The listing builds one solid part. Answer for the finished solid, in the listing's coordinates (mm). A direction names the side the tool comes from. Give positions to 0.01 mm unless a question says otherwise; leave off trailing zeros. Order: outer loops, then holes, each group sorted by start corner. A loop starts at its lowest first (then second) coordinate and runs counter-clockwise, first axis right, second up.
```python
from build123d import *

# Parameters (mm, degrees)
SKETCH1_W                     = 96.825
SKETCH1_H                     = 96.825
BOSS_EXTRUDE1_DEPTH           = 4.7625
FILLET1_R                     = 4
CSK_FOR_M3_SFHCS2_D           = 3.4
CSK_FOR_M3_SFHCS2_CSINK_D     = 6.72
CSK_FOR_M3_SFHCS2_CSINK_ANGLE = 90
CSK_FOR_M3_SFHCS1_D           = 3.4
CSK_FOR_M3_SFHCS1_DEPTH       = 35
CSK_FOR_M3_SFHCS1_CSINK_D     = 6.72
CSK_FOR_M3_SFHCS1_CSINK_ANGLE = 90
CSK_FOR_M3_SFHCS1_TIP         = 1.021463052
M3X0_5_TAPPED_HOLE1_D         = 2.5
M3X0_5_TAPPED_HOLE1_DEPTH     = 10
M3X0_5_TAPPED_HOLE1_TIP       = 0.751075774
M3X0_5_TAPPED_HOLE2_D         = 2.5
M3X0_5_TAPPED_HOLE2_DEPTH     = 10
M3X0_5_TAPPED_HOLE2_TIP       = 0.751075774
M3X0_5_TAPPED_HOLE3_D         = 2.5
M3X0_5_TAPPED_HOLE3_DEPTH     = 10
M3X0_5_TAPPED_HOLE3_TIP       = 0.751075774
M3X0_5_TAPPED_HOLE4_D         = 2.5
M3X0_5_TAPPED_HOLE4_DEPTH     = 10
M3X0_5_TAPPED_HOLE4_TIP       = 0.751075774


with BuildPart() as part:
    # Sketch1 → Boss-Extrude1 (new body, symmetric)
    with BuildSketch(Plane(origin=(0, 0, 0), x_dir=(1, 0, 0), z_dir=(0, 1, 0))):
        Rectangle(SKETCH1_W, SKETCH1_H)
    extrude(amount=BOSS_EXTRUDE1_DEPTH, both=True)

    # Fillet1
    fillet1_edges = [part.edges().sort_by_distance(p)[0] for p in [
        (-48.4125, 0, -48.4125),
        (48.4125, 0, -48.4125),
        (48.4125, 0, 48.4125),
        (-48.4125, 0, 48.4125),
    ]]
    fillet(fillet1_edges, radius=FILLET1_R)

    # CSK for M3 SFHCS2 (through all)
    with Locations(Plane.XZ.offset(4.7625)):
        with Locations((-40, 0), (0, -40), (40, 0), (0, 40)):
            CounterSinkHole(CSK_FOR_M3_SFHCS2_D / 2, CSK_FOR_M3_SFHCS2_CSINK_D / 2, counter_sink_angle=CSK_FOR_M3_SFHCS2_CSINK_ANGLE)

    # CSK for M3 SFHCS1
    with Locations(Plane(origin=(0, 4.7625, 0), x_dir=(1, 0, 0), z_dir=(0, 1, 0))):
        with Locations((-44.4125, 44.4125), (44.4125, 44.4125), (44.4125, -44.4125), (-44.4125, -44.4125)):
            CounterSinkHole(CSK_FOR_M3_SFHCS1_D / 2, CSK_FOR_M3_SFHCS1_CSINK_D / 2, depth=CSK_FOR_M3_SFHCS1_DEPTH, counter_sink_angle=CSK_FOR_M3_SFHCS1_CSINK_ANGLE)
            with Locations((0, 0, -(CSK_FOR_M3_SFHCS1_DEPTH + CSK_FOR_M3_SFHCS1_TIP / 2))):  # 118° drill point
                Cone(0, CSK_FOR_M3_SFHCS1_D / 2, CSK_FOR_M3_SFHCS1_TIP, mode=Mode.SUBTRACT)

    # M3x0.5 Tapped Hole1
    with Locations(Plane.XY.offset(48.4125)):
        with Locations((-30, 0), (30, 0)):
            Hole(M3X0_5_TAPPED_HOLE1_D / 2, depth=M3X0_5_TAPPED_HOLE1_DEPTH)
            with Locations((0, 0, -(M3X0_5_TAPPED_HOLE1_DEPTH + M3X0_5_TAPPED_HOLE1_TIP / 2))):  # 118° drill point
                Cone(0, M3X0_5_TAPPED_HOLE1_D / 2, M3X0_5_TAPPED_HOLE1_TIP, mode=Mode.SUBTRACT)

    # M3x0.5 Tapped Hole2
    with Locations(Plane.ZY.offset(48.4125)):
        with Locations((-30, 0), (30, 0)):
            Hole(M3X0_5_TAPPED_HOLE2_D / 2, depth=M3X0_5_TAPPED_HOLE2_DEPTH)
            with Locations((0, 0, -(M3X0_5_TAPPED_HOLE2_DEPTH + M3X0_5_TAPPED_HOLE2_TIP / 2))):  # 118° drill point
                Cone(0, M3X0_5_TAPPED_HOLE2_D / 2, M3X0_5_TAPPED_HOLE2_TIP, mode=Mode.SUBTRACT)

    # M3x0.5 Tapped Hole3
    with Locations(Plane(origin=(0, 0, -48.4125), x_dir=(-1, 0, 0), z_dir=(0, 0, -1))):
        with Locations((-30, 0), (30, 0)):
            Hole(M3X0_5_TAPPED_HOLE3_D / 2, depth=M3X0_5_TAPPED_HOLE3_DEPTH)
            with Locations((0, 0, -(M3X0_5_TAPPED_HOLE3_DEPTH + M3X0_5_TAPPED_HOLE3_TIP / 2))):  # 118° drill point
                Cone(0, M3X0_5_TAPPED_HOLE3_D / 2, M3X0_5_TAPPED_HOLE3_TIP, mode=Mode.SUBTRACT)

    # M3x0.5 Tapped Hole4
    with Locations(Plane(origin=(48.4125, 0, 0), x_dir=(0, 0, -1), z_dir=(1, 0, 0))):
        with Locations((-30, 0), (30, 0)):
            Hole(M3X0_5_TAPPED_HOLE4_D / 2, depth=M3X0_5_TAPPED_HOLE4_DEPTH)
            with Locations((0, 0, -(M3X0_5_TAPPED_HOLE4_DEPTH + M3X0_5_TAPPED_HOLE4_TIP / 2))):  # 118° drill point
                Cone(0, M3X0_5_TAPPED_HOLE4_D / 2, M3X0_5_TAPPED_HOLE4_TIP, mode=Mode.SUBTRACT)


solid = part.part
```
1) Find section A-A (z = 0). Write down the section's boundary in (x, y).
Geometry says:
outline: (-48.41, -4.76) - (-43.36, -4.76) - (-41.7, -3.1) - (-41.7, 4.76) - (-48.41, 4.76) - close; (-38.3, -3.1) - (-36.64, -4.76) - (36.64, -4.76) - (38.3, -3.1) - (38.3, 4.76) - (-38.3, 4.76) - close; (41.7, -3.1) - (43.36, -4.76) - (48.41, -4.76) - (48.41, 4.76) - (41.7, 4.76) - close
2) For a pull along Z with two mould halves and no side action, classify faces 1 (the flat face through (48.412, 0, 1)), 2 (the cylindrical face through (-47.27, -0.07, -47.21)), 3 (the flat face through (-1, 0, 48.412)), 4 (the conical face through (-37.79, -0.08, -29.8)) as +Z half, -Z half, draft (parallel to the pull), parting line (faces both ways), or undercut.
Geometry says:
face 1: draft
face 2: -Z half
face 3: +Z half
face 4: undercut
3) Given P1, Ø2, axis at x = 30, y = 0, coming from the +Z side; P2, Ø2, axis at x = -30, y = 0, coming from the -Z side; P3, Ø1.5, axis at y = 0, z = 30, coming from the +X side, each flat-ended and moving along its own axis, determine where each tip first touches the part or whether it passes through.
Geometry says:
P1: stops at z = 38.26
P2: stops at z = -38.26
P3: stops at x = 38.11
4) Straight lines are drawn through the part: probe 1 along X at (y, z) = (0, 42.25); probe 2 along Y at (x, z) = (42, -30); probe 3 along Z at (x, y) = (40, -0.75). For each, find the intervals that lie inside material, in ascending order.
Geometry says:
probe 1: x = -48.41 to -31.25, -28.75 to 28.75, 31.25 to 48.41
probe 2: y = -4.76 to -1.25, 1.25 to 4.76
probe 3: z = -48.41 to -31, -29 to -1.7, 1.7 to 29, 31 to 48.41
5) A tool of negligible diameter and unlimited length cuts with its end or side. For faces 5 (the cylindrical face through (31.155, -0.479, -43.342)), 6 (the cylindrical face through (-43.342, -0.479, -31.155)), 7 (the cylindrical face through (43.342, -0.479, 31.155)), 8 (the cylindrical face through (-31.155, -0.479, 43.342)), from which of +Z, -Z, +X, -X, +Y, -Y can it reach the whole face along a straight path? Write none if from no direction.
Geometry says:
face 5: -Z
face 6: -X
face 7: +X
face 8: +Z
